```python
from build123d import *

# Parameters (mm, degrees)
SKETCH3_R           = 30
BOSS_EXTRUDE3_DEPTH = 2
BOSS_EXTRUDE4_DEPTH = 15
CUT_EXTRUDE1_DEPTH  = 10


with BuildPart() as part:
    # Sketch3 → Boss-Extrude3 (new body)
    with BuildSketch(Plane(origin=(0, 0, 0), x_dir=(1, 0, 0), z_dir=(0, 1, 0))):
        with Locations(Location((0, 0, 0), (0, 0, 270))):
            Circle(SKETCH3_R)
    extrude(amount=BOSS_EXTRUDE3_DEPTH)

    # Sketch4 → Boss-Extrude4 (add)
    with BuildSketch(Plane(origin=(0, 2, 0), x_dir=(1, 0, 0), z_dir=(0, 1, 0))):
        with BuildLine():
            Line((14.638601317, -17.740105735), (19.093827805, -23.13926835))
            ThreePointArc((19.093827805, -23.13926835), (26.293545079, -14.444704468), (29.770348498, -3.704908943))
            Line((29.770348498, -3.704908943), (22.823933849, -2.84043019))
            ThreePointArc((22.823933849, -2.84043019), (20.158384561, -11.074273425), (14.638601317, -17.740105735))
        make_face()
        with BuildLine():
            Line((21.39541974, 8.440143018), (27.907069226, 11.008882197))
            ThreePointArc((27.907069226, 11.008882197), (21.862882582, 20.542988225), (12.723121407, 27.168404106))
            Line((12.723121407, 27.168404106), (9.754393079, 20.829109814))
            ThreePointArc((9.754393079, 20.829109814), (16.761543313, 15.749624306), (21.39541974, 8.440143018))
        make_face()
        with BuildLine():
            Line((-1.415504714, 22.95640099), (-1.846310497, 29.943131726))
            ThreePointArc((-1.846310497, 29.943131726), (-12.781540551, 27.140969421), (-21.907027026, 20.495906101))
            Line((-21.907027026, 20.495906101), (-16.795387386, 15.713528011))
            ThreePointArc((-16.795387386, 15.713528011), (-9.799181089, 20.808076556), (-1.415504714, 22.95640099))
        make_face()
        with BuildLine():
            Line((-22.270249764, 5.747693053), (-29.048151867, 7.496990939))
            ThreePointArc((-29.048151867, 7.496990939), (-29.762309071, -3.768946635), (-26.262408702, -14.501237505))
            Line((-26.262408702, -14.501237505), (-20.134513338, -11.117615421))
            ThreePointArc((-20.134513338, -11.117615421), (-22.817770288, -2.889525753), (-22.270249764, 5.747693053))
        make_face()
        with BuildLine():
            Line((-12.348266578, -19.404131326), (-16.106434667, -25.309736512))
            ThreePointArc((-16.106434667, -25.309736512), (-5.612578038, -29.470306543), (5.675965822, -29.458163758))
            Line((5.675965822, -29.458163758), (4.351573797, -22.584592214))
            ThreePointArc((4.351573797, -22.584592214), (-4.302976496, -22.593901683), (-12.348266578, -19.404131326))
        make_face()
    extrude(amount=BOSS_EXTRUDE4_DEPTH)

    # Sketch5 → Cut-Extrude1 (cut)
    with BuildSketch(Plane.XZ):
        Polygon((7.002775602, -0.757936148), (4.157779759, 5.685613494), (-2.844995843, 6.443549642), (-7.002775602, 0.757936148), (-4.157779759, -5.685613494), (2.844995843, -6.443549642), align=None)
    extrude(amount=-CUT_EXTRUDE1_DEPTH, mode=Mode.SUBTRACT)


solid = part.part
```
Input: part model. Units: mm. Frame: model coordinates. A direction names the side the tool comes from. Coordinates: 2 decimals unless noted, no trailing zeros. Loops run counter-clockwise (first coordinate to the right, second up) from the corner with the lowest first, then second, coordinate; pieces in that order, holes last. Notation, with made-up numbers: (-0.75, -29) -> (11.25, -29) arc R32 cw to (11.25, 2) -> close; hole circle Ø7 at (77, 17). An arc over 180 degrees is marked (long way). Use a Markdown table: item, result.
1) Pull-direction query (X, two-part tool) for faces 6 (the flat face through (0.71, 0.99, 6.06)), 7 (the flat face through (-26, 17, 3)), 8 (the flat face through (-25.61, 9.4, -6.61)); classes: released by +X, released by -X, zero draft, split by the parting line, or undercut.
Results found:
| item | result |
|---|---|
| face 6 | undercut |
| face 7 | zero draft |
| face 8 | released by +X |
2) Material intervals for line 1 along Z through (x, y) = (16.5, 4.25); line 2 along X through (y, z) = (4.5, 6); line 3 along Y through (x, z) = (-8.5, -20), sorted ascending. Write a range as from..to.
Results found:
| item | result |
|---|---|
| line 1 | z = -25.05..-16.02, 16.02..20 |
| line 2 | x = -29.39..-22.2, 22.2..29.39 |
| line 3 | y = 0..2 |
3) Cut plane A-A (y = 11.25). Return the cut outline in (x, z), then the cut area to 3 significant figures.
Results found:
| item | result |
|---|---|
| outline | (-29.05, -7.5) -> (-22.27, -5.75) arc R23 cw to (-20.13, 11.12) -> (-26.26, 14.5) arc R30 ccw to start; (-21.91, -20.5) arc R30 ccw to (-1.85, -29.94) -> (-1.42, -22.96) arc R23 cw to (-16.8, -15.71) -> close; (-16.11, 25.31) -> (-12.35, 19.4) arc R23 cw to (4.35, 22.58) -> (5.68, 29.46) arc R30 ccw to start; (9.75, -20.83) -> (12.72, -27.17) arc R30 ccw to (27.91, -11.01) -> (21.4, -8.44) arc R23 cw to start; (14.64, 17.74) arc R23 cw to (22.82, 2.84) -> (29.77, 3.7) arc R30 ccw to (19.09, 23.14) -> close |
| area | 702 mm2 |
4) Cut plane C-C (x = -18). Return the cut outline in (y, z).
Results found:
| item | result |
|---|---|
| outline | (0, -24) -> (17, -24) -> (17, -16.84) -> (2, -16.84) -> (2, 24) -> (0, 24) -> close |
5) Contact query for flat-ended pins moving along their axis: pin 1 (4 mm diameter, centred on x = -3.5, y = 6.5, fed in from -Z); pin 2 (4 mm diameter, centred on x = -13, y = 10.5, fed in from +Z); pin 3 (3 mm diameter, centred on x = 7.5, y = 2.5, fed in from -Z). Output: stop coordinate, or through.
Results found:
| item | result |
|---|---|
| pin 1 | stops at z = -29.94 |
| pin 2 | stops at z = 27.91 |
| pin 3 | stops at z = -29.38 |
6) Access query for faces 1 (the flat face through (-19.39, 9.4, -18.14)), 2 (the flat face through (16.835, 9.395, 20.402)), 3 (the flat face through (11.26, 9.4, -24.04)), 4 (the flat face through (-5.6, 0.99, -2.42)), 5 (the cylindrical face through (16.678, 9.395, -15.838)). Directions: +Z, -Z, +X, -X, +Y, -Y. A direction counts if a zero-diameter tool reaches every point of the face in a straight line with its end or side. Return the directions, or none.
Results found:
| item | result |
|---|---|
| face 1 | -X, +Y |
| face 2 | +Z, +Y |
| face 3 | -Z, +Y |
| face 4 | +Y, -Y |
| face 5 | +Y |
7) Cut plane D-D (x = 0). Return the cut outline in (y, z), then the cut area to 3 significant figures.
Results found:
| item | result |
|---|---|
| outline | (0, -30) -> (2, -30) -> (2, -6.14) -> (0, -6.14) -> close; (0, 6.14) -> (2, 6.14) -> (2, 23) -> (17, 23) -> (17, 30) -> (0, 30) -> close |
| area | 200 mm2 |
8) Cut plane B-B (z = -2.5). Return the cut outline in (x, y), then the cut area to 3 significant figures.
Results found:
| item | result |
|---|---|
| outline | (-29.9, 0) -> (-5.56, 0) -> (-5.56, 2) -> (-22.86, 2) -> (-22.86, 17) -> (-29.9, 17) -> close; (5.73, 0) -> (29.9, 0) -> (29.9, 2) -> (5.73, 2) -> close |
| area | 202 mm2 |
